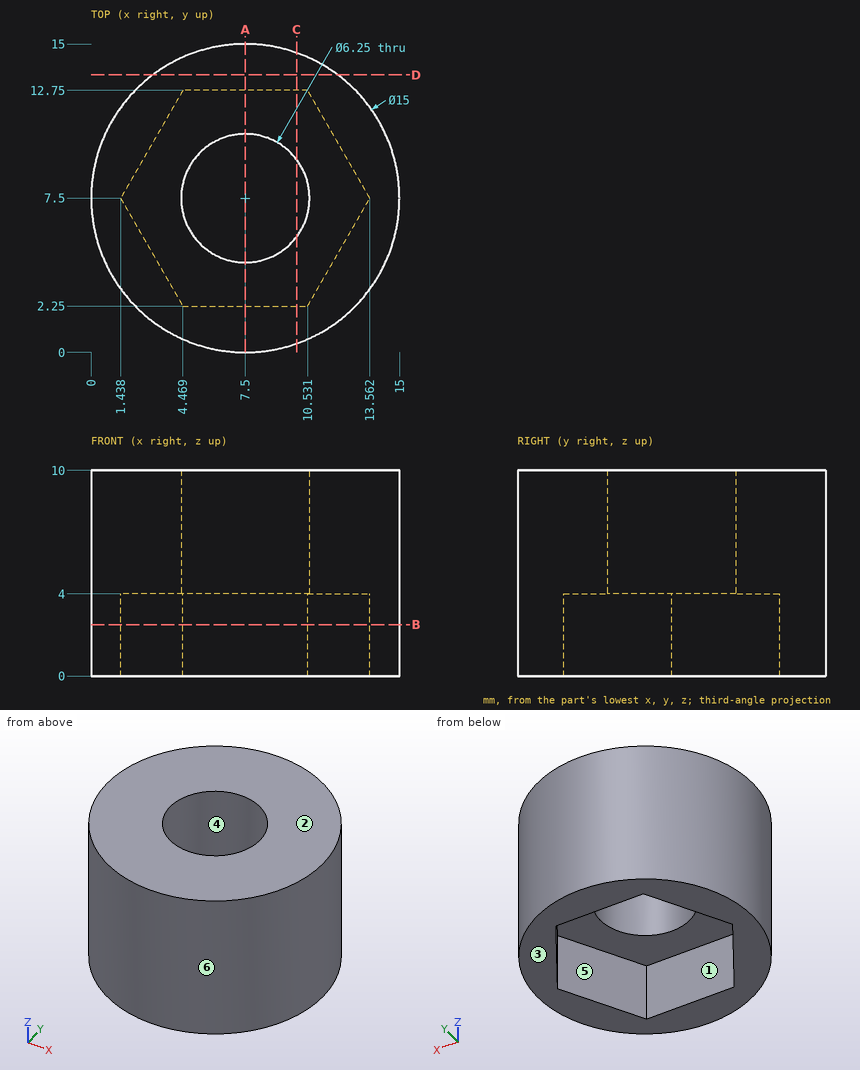
For this review, use the dimensioned drawing (mm, ordinates from the lowest corner) and the shaded views. A direction names the side the tool comes from. Give positions to 0.01 mm unless a question says otherwise; leave off trailing zeros. Order: outer loops, then holes, each group sorted by start corner. A loop starts at its lowest first (then second) coordinate and runs counter-clockwise, first axis right, second up.
1. Mouldability with a two-part tool opening along Y and no side actions: class the marked faces 3, 4, 5 and 6 as +Y half, -Y half, draft (parallel to the pull), parting line (faces both ways), or undercut.
Solution:
face 3: draft
face 4: undercut
face 5: undercut
face 6: parting line
2. Add section C-C, the plane x = 10. State the section outline as (y, z) points (3 decimals), then the cut area to 3 significant figures.
Solution:
outline: (0.429, 0) - (2.25, 0) - (2.25, 4) - (5.625, 4) - (5.625, 10) - (0.429, 10) - close; (9.375, 4) - (12.75, 4) - (12.75, 0) - (14.571, 0) - (14.571, 10) - (9.375, 10) - close
area: 76.9 mm2
3. To check wall thickness, follow L1, parallel to Y at x = 7.5, z = 5.7 (3 decimals); L2, parallel to Y at x = 2, z = 1.25 (1 decimal); L3, parallel to Z at x = 11.5, y = 4.25. State the ranges of each line that lie inside material, in increasing order.
Solution:
L1: y = 0 to 4.375, 10.625 to 15
L2: y = 2.4 to 6.5, 8.5 to 12.6
L3: z = 4 to 10
4. Tool access review of the marked faces 1 and 2: name each direction out of +Z, -Z, +X, -X, +Y, -Y from which nothing blocks a thin tool from reaching the whole face with its end or side.
Solution:
face 1: -Z
face 2: +Z, +X, -X, +Y, -Y
5. Add section A-A, the plane x = 7.5. State the section outline as (y, z) points (3 decimals), then the cut area to 3 significant figures.
Solution:
outline: (0, 0) - (2.25, 0) - (2.25, 4) - (4.375, 4) - (4.375, 10) - (0, 10) - close; (10.625, 4) - (12.75, 4) - (12.75, 0) - (15, 0) - (15, 10) - (10.625, 10) - close
area: 70.5 mm2
6. For pin 1 Ø3 at (x, y) = (5.5, 10) entering from -Z; pin 2 Ø1.5 at (x, z) = (9, 3) entering from -Y; pin 3 Ø3 at (x, y) = (12.5, 6) entering from -Z; pin 4 Ø2 at (x, z) = (11, 8.5) entering from +Y, all flat-tipped, find the tip position at first contact; note any pin that passes through.
Solution:
pin 1: stops at z = 4
pin 2: stops at y = 0.04
pin 3: stops at z = 0
pin 4: stops at y = 14.57
7. Add section B-B, the plane z = 2.5. State the section outline as (x, y) points.
Solution:
outline: circle Ø15 at (7.5, 7.5); hole (1.44, 7.5) - (4.47, 2.25) - (10.53, 2.25) - (13.56, 7.5) - (10.53, 12.75) - (4.47, 12.75) - close
8. Add section D-D, the plane y = 13.5. State the section outline as (x, z) points, then the cut area to 3 significant figures.
Solution:
outline: (3, 0) - (12, 0) - (12, 10) - (3, 10) - close
area: 90.0 mm2
